Could you check a few things on this model? Use its own coordinates, in mm. Face numbers are marked on the shaded views. Give positions to 0.01 mm unless a question says otherwise; leave off trailing zeros. Loops run counter-clockwise (first coordinate to the right, second up) from the corner with the lowest first, then second, coordinate; pieces in that order, holes last. Notation, with made-up numbers: (39, 50) - (60, 50) arc R13 cw to (60, 71) - close; hole circle Ø7 at (-11, 61.25). An arc over 180 degrees is marked (long way). One line per item, written item: value. Start each with the question number.
Q1. If I drill on line 1 (Y direction, x = 0, z = 30.8); line 2 (Z direction, x = -0.5, y = -22.5); line 3 (X direction, y = 24.71, z = 30.7), over which ranges is the centre line in solid material (lowest first)? Write a range as from..to.
Q2. I want a section at A-A (y = -24.71). Please give me the cut outline in (x, z).
Q3. I'm going to push flat-ended pins straight in: P1, Ø1, axis at x = 2.5, z = -5.5, coming from the -Y side; P2, Ø1, axis at x = 0.5, z = 7, coming from the +Y side. Where does each tip first touch, or does it pass through?
Q4. If we mould it in two halves opening along Z, with no side actions, what happens to the marked faces 1, 2, 3 and 4? For each: released by +Z, released by -Z, zero draft, split by the parting line, or undercut.
Q5. I want a section at C-C (z = 27). Please give me the cut outline in (x, y), then the cut area to 3 significant figures.
```python
from build123d import *

# Parameters (mm, degrees)
SKETCH_1_W          = 8
SKETCH_1_H          = 60
SKETCH_1_R          = 1.8
EXTRUDE_1_DEPTH     = 32
SKETCH_2_W          = 56
SKETCH_2_H          = 12
CUT_EXTRUDE_1_DEPTH = 30


with BuildPart() as part:
    # Sketch 1 → Extrude 1 (new, symmetric)
    with BuildSketch(Plane.XY):
        Rectangle(SKETCH_1_W, SKETCH_1_H)
        with Locations((0, 24.71)):
            Circle(SKETCH_1_R, mode=Mode.SUBTRACT)
        with Locations(Location((0, -24.71, 0), (0, 0, 180))):
            Circle(SKETCH_1_R, mode=Mode.SUBTRACT)
    extrude(amount=EXTRUDE_1_DEPTH, both=True)

    # Sketch 2 → Cut-Extrude 1 (cut)
    with BuildSketch(Plane.ZY.offset(4)):
        with Locations((0, 24)):
            Rectangle(SKETCH_2_W, SKETCH_2_H)
        with Locations((0, -24)):
            Rectangle(SKETCH_2_W, SKETCH_2_H)
    extrude(amount=-CUT_EXTRUDE_1_DEPTH, mode=Mode.SUBTRACT)


solid = part.part
```
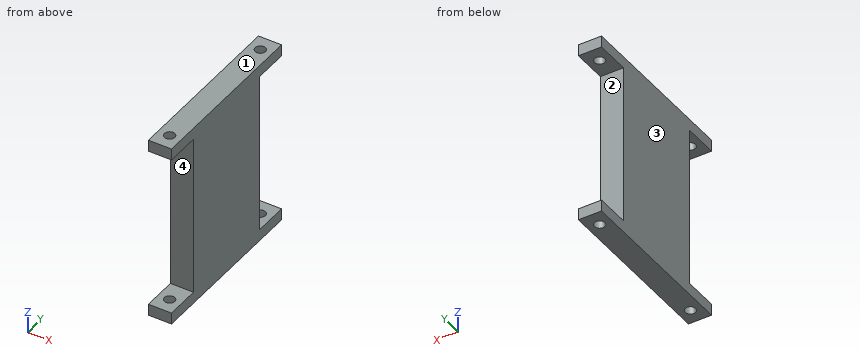
Worked answers:
1. line 1: y = -30..-26.51, -22.91..22.91, 26.51..30
1. line 2: z = -32..-28, 28..32
1. line 3: x = -4..-1.8, 1.8..4
2. outline: (-4, -32) - (-1.8, -32) - (-1.8, -28) - (-4, -28) - close; (-4, 28) - (-1.8, 28) - (-1.8, 32) - (-4, 32) - close; (1.8, -32) - (4, -32) - (4, -28) - (1.8, -28) - close; (1.8, 28) - (4, 28) - (4, 32) - (1.8, 32) - close
3. P1: stops at y = -18
3. P2: stops at y = 18
4. face 1: released by +Z
4. face 2: undercut
4. face 3: zero draft
4. face 4: undercut
5. outline: (-4, -18) - (4, -18) - (4, 18) - (-4, 18) - close
5. area: 288 mm²
